The listing builds one solid part. Answer for the finished solid, in the listing's coordinates (mm). A direction names the side the tool comes from. Round coordinates to 2 decimals unless told otherwise and drop trailing zeros. Order: outer loops, then holes, each group sorted by start corner. A loop starts at its lowest first (then second) coordinate and runs counter-clockwise, first axis right, second up. Notation, with made-up numbers: (28.5, 62.25) - (69.5, 62.25) arc R16 ccw to (69.5, 68.25) - close; hole circle Ø2 at (57, 6). An arc over 180 degrees is marked (long way). One line per item, written item: value. Start each with the question number.
1. Straight lines are drawn through the part: line 1 (Y direction, x = -9.5, z = -28.75); line 2 (Z direction, x = -17.5, y = -3); line 3 (Y direction, x = -27, z = -30). For each, find the intervals that lie inside material, in ascending order.
2. Flat-ended cylindrical pins translate along their axes: P1, Ø10, axis at x = -10, y = -47, coming from the -Z side; P2, Ø22.5, axis at x = -9.5, y = -47, coming from the -Z side; P3, Ø4, axis at x = 0, y = -23, coming from the +Z side; P4, Ø1.5, axis at x = -8.5, z = -28.5, coming from the +Y side. Find the tip coordinate at first contact, or state that the pin passes through.
3. Section C-C, the plane x = -9.5 is taken. Give the vertices of the cut face in (y, z), then the cut area to 3 significant figures.
4. Section D-D, the plane y = 2 is taken. Give the vertices of the cut face in (x, z).
5. Section B-B, the plane x = -19 is taken. Give the vertices of the cut face in (y, z).
6. For a pull along Y with two mould halves and no side action, classify faces 4 (the flat face through (0, -53, -7.5)), 5 (the flat face through (0, -23, -27.08)), 6 (the flat face through (-17, 10, -30)) as released by +Y, released by -Y, zero draft, split by the parting line, or undercut.
7. Section A-A, the plane y = -55 is taken. Give the vertices of the cut face in (x, z), then the cut area to 3 significant figures.
8. A tool of negligible diameter and unlimited length cuts with its end or side. For faces 1 (the flat face through (-16, 0, 27.5)), 2 (the flat face through (-22.5, -48, -30)), 3 (the flat face through (-16, -50, -32.08)), from which of +Z, -Z, +X, -X, +Y, -Y can it reach the whole face along a straight path? Write none if from no direction.
from build123d import *

# Parameters (mm, degrees)
BOSS_EXTRUDE1_DEPTH      = 2.5
BOSS_EXTRUDE1_DEPTH_BACK = 2.5
SKETCH2_R                = 2.5
CUT_EXTRUDE1_DEPTH       = 67.01762189
BOSS_EXTRUDE2_DEPTH      = 2.5
BOSS_EXTRUDE2_DEPTH_BACK = 2.5
SKETCH3_W                = 65
SKETCH3_H                = 20
SKETCH5_W                = 5
SKETCH5_H                = 20
BOSS_EXTRUDE4_DEPTH      = 35
SKETCH6_R                = 7
CUT_EXTRUDE2_DEPTH       = 97.079394253
SKETCH7_W                = 15
SKETCH7_H                = 15
CUT_EXTRUDE3_DEPTH       = 77.689308251
SKETCH8_W                = 25
SKETCH8_H                = 24
BOSS_EXTRUDE5_DEPTH      = 5
CUT_EXTRUDE4_DEPTH       = 93.498791343
CUT_EXTRUDE4_DEPTH_BACK  = 93.498791343
SKETCH9_R                = 7


with BuildPart() as part:
    # Sketch1 → Boss-Extrude1 (new, two sides: drawn at the far end of the back side and taken through both)
    with BuildSketch(Plane(origin=(0, 0, 0), x_dir=(0, 0, -1), z_dir=(1, 0, 0)).offset(-BOSS_EXTRUDE1_DEPTH_BACK)):
        with BuildLine():
            Line((-27.08, 0), (-27.08, -60))
            Line((-27.08, -60), (27.08, -60))
            Line((27.08, -60), (27.08, 0))
            ThreePointArc((27.08, 0), (0, 27.08), (-27.08, 0))
        make_face()
    extrude(amount=BOSS_EXTRUDE1_DEPTH + BOSS_EXTRUDE1_DEPTH_BACK)

    # Sketch2 → Cut-Extrude1 (cut, through all)
    with BuildSketch(Plane(origin=(2.5, 0, 0), x_dir=(0, 0, -1), z_dir=(1, 0, 0))):
        with Locations((-14.142135624, 14.142135624)):
            Circle(SKETCH2_R)
        with Locations((14.142135624, 14.142135624)):
            Circle(SKETCH2_R)
        with Locations((14.142135624, -14.142135624)):
            Circle(SKETCH2_R)
        with Locations((-14.142135624, -14.142135624)):
            Circle(SKETCH2_R)
    extrude(amount=-CUT_EXTRUDE1_DEPTH, mode=Mode.SUBTRACT)

    # Sketch3 → Boss-Extrude2 (add, two sides: drawn at the far end of the back side and taken through both)
    with BuildSketch(Plane(origin=(0, 0, 0), x_dir=(0, 0, -1), z_dir=(1, 0, 0)).offset(-BOSS_EXTRUDE2_DEPTH_BACK)):
        Rectangle(SKETCH3_W, SKETCH3_H)
    extrude(amount=BOSS_EXTRUDE2_DEPTH + BOSS_EXTRUDE2_DEPTH_BACK)

    # Sketch5 → Boss-Extrude4 (add)
    with BuildSketch(Plane.ZY.offset(2.5)):
        with Locations((-30, 0)):
            Rectangle(SKETCH5_W, SKETCH5_H)
        with Locations((30, 0)):
            Rectangle(SKETCH5_W, SKETCH5_H)
    extrude(amount=BOSS_EXTRUDE4_DEPTH)

    # Sketch6 → Cut-Extrude2 (cut, through all)
    with BuildSketch(Plane(origin=(0, 0, -32.5), x_dir=(-1, 0, 0), z_dir=(0, 0, -1))):
        with Locations((27.5, 0)):
            Circle(SKETCH6_R)
    extrude(amount=-CUT_EXTRUDE2_DEPTH, mode=Mode.SUBTRACT)

    # Sketch7 → Cut-Extrude3 (cut, through all)
    with BuildSketch(Plane.ZY.offset(2.5)):
        with Locations((0, -52.5)):
            Rectangle(SKETCH7_W, SKETCH7_H)
    extrude(amount=-CUT_EXTRUDE3_DEPTH, mode=Mode.SUBTRACT)

    # Sketch8 → Boss-Extrude5 (add)
    with BuildSketch(Plane.XY.offset(27.08)):
        with Locations((-10, -48)):
            Rectangle(SKETCH8_W, SKETCH8_H)
    boss_extrude5 = extrude(amount=BOSS_EXTRUDE5_DEPTH)

    # Mirror1: Boss-Extrude5 across plane
    add(boss_extrude5.mirror(Plane.XY))

    # Sketch9 → Cut-Extrude4 (cut, two sides: drawn at the far end of the back side and taken through both)
    with BuildSketch(Plane(origin=(0, 0, 27.08), x_dir=(-1, 0, 0), z_dir=(0, 0, -1)).offset(-CUT_EXTRUDE4_DEPTH_BACK)):
        with Locations((9.5, -47)):
            Circle(SKETCH9_R)
    extrude(amount=CUT_EXTRUDE4_DEPTH + CUT_EXTRUDE4_DEPTH_BACK, mode=Mode.SUBTRACT)


solid = part.part
Answer list:
1. line 1: y = -60 to -54, -40 to -36, -10 to 10
1. line 2: z = -32.5 to -27.5, 27.5 to 32.5
1. line 3: y = -10 to -6.98, 6.98 to 10
2. P1: passes through
2. P2: stops at z = -32.08
2. P3: stops at z = 27.08
2. P4: stops at y = 10
3. outline: (-60, -32.08) - (-54, -32.08) - (-54, -27.08) - (-60, -27.08) - close; (-60, 27.08) - (-54, 27.08) - (-54, 32.08) - (-60, 32.08) - close; (-40, -32.08) - (-36, -32.08) - (-36, -27.08) - (-40, -27.08) - close; (-40, 27.08) - (-36, 27.08) - (-36, 32.08) - (-40, 32.08) - close; (-10, -32.5) - (10, -32.5) - (10, -27.5) - (-10, -27.5) - close; (-10, 27.5) - (10, 27.5) - (10, 32.5) - (-10, 32.5) - close
3. area: 300 mm²
4. outline: (-37.5, -32.5) - (-34.21, -32.5) - (-34.21, -27.5) - (-37.5, -27.5) - close; (-37.5, 27.5) - (-34.21, 27.5) - (-34.21, 32.5) - (-37.5, 32.5) - close; (-20.79, -32.5) - (2.5, -32.5) - (2.5, 32.5) - (-20.79, 32.5) - (-20.79, 27.5) - (-2.5, 27.5) - (-2.5, -27.5) - (-20.79, -27.5) - close
5. outline: (-60, -32.08) - (-36, -32.08) - (-36, -27.08) - (-60, -27.08) - close; (-60, 27.08) - (-36, 27.08) - (-36, 32.08) - (-60, 32.08) - close; (-10, -32.5) - (10, -32.5) - (10, -27.5) - (-10, -27.5) - close; (-10, 27.5) - (10, 27.5) - (10, 32.5) - (-10, 32.5) - close
6. face 4: zero draft
6. face 5: undercut
6. face 6: released by +Y
7. outline: (-22.5, -32.08) - (2.5, -32.08) - (2.5, -7.5) - (-2.5, -7.5) - (-2.5, -27.08) - (-22.5, -27.08) - close; (-22.5, 27.08) - (-2.5, 27.08) - (-2.5, 7.5) - (2.5, 7.5) - (2.5, 32.08) - (-22.5, 32.08) - close
7. area: 446 mm²
8. face 1: -X, +Y
8. face 2: +Z, -Z, -X, -Y
8. face 3: -Z, +X, -X, -Y
